The figure shows three views and two pictorial views of one solid part (mm, origin at its lowest corner). Answer the questions. Coordinates: 2 decimals unless noted, no trailing zeros. Order: outer loops, then holes, each group sorted by start corner. A loop starts at its lowest first (then second) coordinate and runs counter-clockwise, first axis right, second up. Notation, with made-up numbers: (59.25, 26) -> (91.25, 26) arc R20 cw to (91.25, 47) -> close; hole circle Ø10 at (72, 60.5). An arc over 180 degrees is marked (long way). Write item = value, one per line. Start each with the question number.
Q1. The part is cut by section C-C, the plane y = 38.1. Determine the outline of the cut face in (x, z) (1 decimal).
Q2. Flat-ended cylindrical pins translate along their axes: pin 1 (3 mm diameter, centred on x = 9.5, z = 1.5, fed in from +Y); pin 2 (9 mm diameter, centred on x = 12.7, y = 63.5, fed in from -Z). Find the tip coordinate at first contact, or state that the pin passes through.
Q3. The part is cut by section A-A, the plane z = 6.5. Count the separate pieces of the cut face and the enclosed holes in it, plus the area to 3 significant figures.
Q4. The part is cut by section D-D, the plane x = 23.25. Determine the outline of the cut face in (y, z) (1 decimal).
Q5. For a pull along X with two mould halves and no side action, classify the marked faces 1, 2, 3 and 4 as +X half, -X half, draft (parallel to the pull), parting line (faces both ways), or undercut.
Q6. Straight lines are drawn through the part: L1, parallel to Y at x = 13, z = 5.5 (1 decimal); L2, parallel to Y at x = 12.7, z = 3; L3, parallel to Y at x = 12.7, z = 8.75. For each, find the intervals that lie inside material, in ascending order. Write a range as from..to.
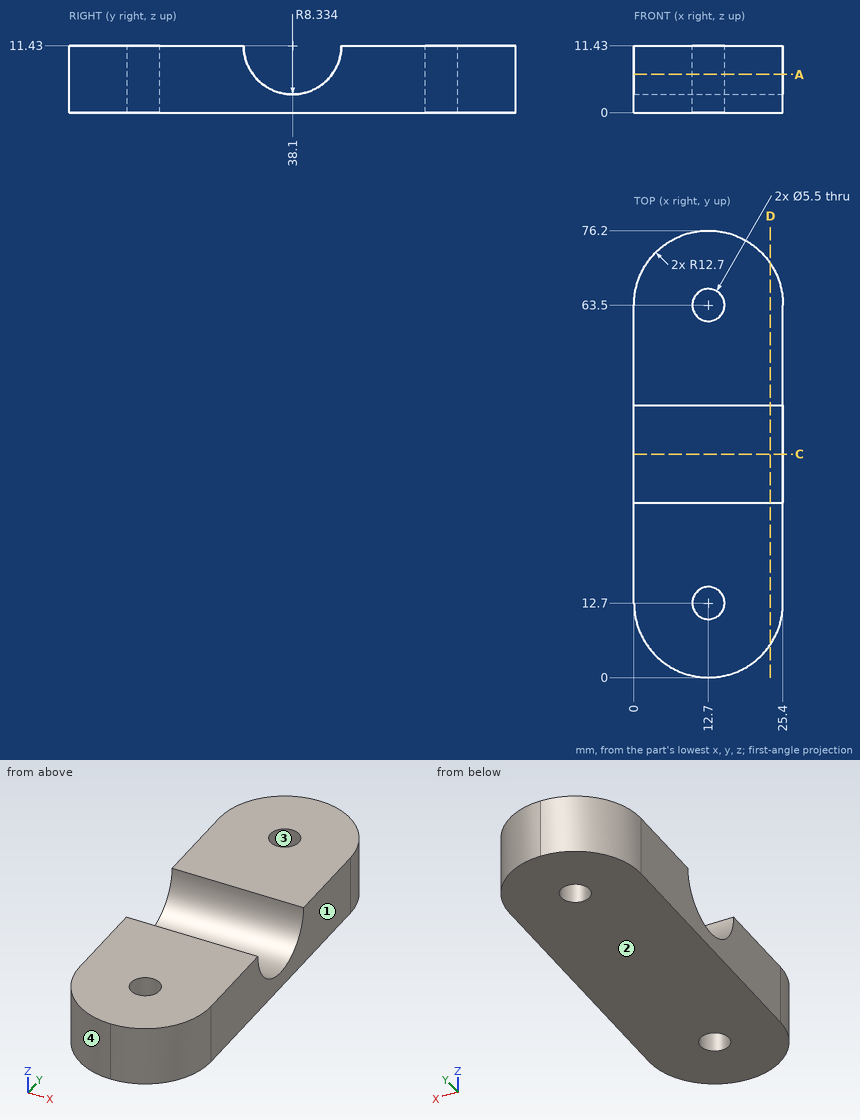
Model answer:
q1.outline = (0, 0) -> (25.4, 0) -> (25.4, 3.1) -> (0, 3.1) -> close
q2.pin_1 = 76.09
q2.pin_2 = 0
q3.separate_pieces = 2
q3.enclosed_holes = 2
q3.area = 1,410 mm2
q4.outline = (5.6, 0) -> (70.6, 0) -> (70.6, 11.4) -> (46.4, 11.4) arc R8.3 cw to (29.8, 11.4) -> (5.6, 11.4) -> close
q5.face_1 = +X half
q5.face_2 = draft
q5.face_3 = undercut
q5.face_4 = -X half
q6.L1 = 0..10, 15.4..32.2, 44..60.8, 66.2..76.2
q6.L2 = 0..9.95, 15.45..60.75, 66.25..76.2
q6.L3 = 0..9.95, 15.45..30.21, 45.99..60.75, 66.25..76.2
